CAD build for the part. Positions are in the model's coordinates, mm. Face numbers are marked on the shaded views. A direction names the side the tool comes from. Round coordinates to 2 decimals unless told otherwise and drop trailing zeros. Loops run counter-clockwise (first coordinate to the right, second up) from the corner with the lowest first, then second, coordinate; pieces in that order, holes last. Notation, with made-up numbers: (58.25, -6) - (103.25, -6) arc R10 cw to (103.25, 1) - close; hole circle Ø9 at (69.5, 11.5). An arc over 180 degrees is marked (long way). One line per question, with ' | ' between items.
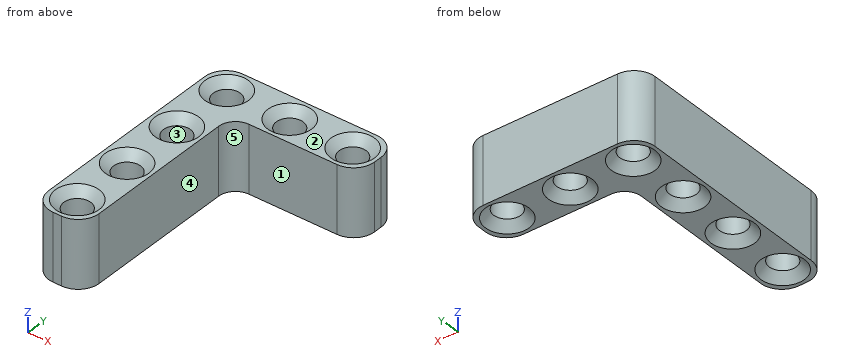
```python
from build123d import *

# Parameters (mm, degrees)
SKETCH1_R           = 1.6
BOSS_EXTRUDE1_DEPTH = 8
CHAMFER1_SIZE       = 1
SKETCH2_R           = 1.6
BOSS_EXTRUDE3_DEPTH = 8
FILLET1_R           = 2
CHAMFER5_SIZE       = 1


with BuildPart() as part:
    # Sketch1 → Boss-Extrude1 (new body)
    with BuildSketch(Plane.XY):
        with BuildLine():
            Line((-0.5, 3), (15.5, 3))
            ThreePointArc((15.5, 3), (17.267766953, 2.267766953), (18, 0.5))
            Line((18, 0.5), (18, -0.5))
            ThreePointArc((18, -0.5), (17.267766953, -2.267766953), (15.5, -3))
            Line((15.5, -3), (-0.5, -3))
            ThreePointArc((-0.5, -3), (-2.267766953, -2.267766953), (-3, -0.5))
            Line((-3, -0.5), (-3, 0.5))
            ThreePointArc((-3, 0.5), (-2.267766953, 2.267766953), (-0.5, 3))
        make_face()
        Circle(SKETCH1_R, mode=Mode.SUBTRACT)
        with Locations((7.5, 0)):
            Circle(SKETCH1_R, mode=Mode.SUBTRACT)
        with Locations((15, 0)):
            Circle(SKETCH1_R, mode=Mode.SUBTRACT)
    extrude(amount=BOSS_EXTRUDE1_DEPTH)

    # Chamfer1
    chamfer1_edges = [part.edges().sort_by_distance(p)[0] for p in [
        (-1.6, 0, 0),
        (-1.6, 0, 8),
        (5.9, 0, 0),
        (5.9, 0, 8),
        (13.4, 0, 0),
        (13.4, 0, 8),
    ]]
    chamfer(chamfer1_edges, length=CHAMFER1_SIZE)

    # Sketch2 → Boss-Extrude3 (add)
    with BuildSketch(Plane.XY.offset(8)):
        with BuildLine():
            ThreePointArc((-0.5, -3), (-2.267766953, -2.267766953), (-3, -0.5))
            Line((-3, -0.5), (-3, -23))
            ThreePointArc((-3, -23), (-2.267766953, -24.767766953), (-0.5, -25.5))
            Line((-0.5, -25.5), (0.5, -25.5))
            ThreePointArc((0.5, -25.5), (2.267766953, -24.767766953), (3, -23))
            Line((3, -23), (3, -3))
            Line((3, -3), (-0.5, -3))
        make_face()
        with Locations((0, -22.5)):
            Circle(SKETCH2_R, mode=Mode.SUBTRACT)
        with Locations((0, -15)):
            Circle(SKETCH2_R, mode=Mode.SUBTRACT)
        with Locations((0, -7.5)):
            Circle(SKETCH2_R, mode=Mode.SUBTRACT)
    extrude(amount=-BOSS_EXTRUDE3_DEPTH)

    # Fillet1
    fillet1_edges = [part.edges().sort_by_distance(p)[0] for p in [
        (3, -3, 4),
    ]]
    fillet(fillet1_edges, radius=FILLET1_R)

    # Chamfer5
    chamfer5_edges = [part.edges().sort_by_distance(p)[0] for p in [
        (-1.6, -7.5, 8),
        (-1.6, -15, 8),
        (-1.6, -22.5, 8),
        (-1.6, -22.5, 0),
        (-1.6, -15, 0),
        (-1.6, -7.5, 0),
    ]]
    chamfer(chamfer5_edges, length=CHAMFER5_SIZE)


solid = part.part
```
(1) Cut at B-B, the plane z = 1.5. Write the cut outline in (x, y).
Results found:
outline: (-3, -23) arc R2.5 ccw to (-0.5, -25.5) - (0.5, -25.5) arc R2.5 ccw to (3, -23) - (3, -5) arc R2 cw to (5, -3) - (15.5, -3) arc R2.5 ccw to (18, -0.5) - (18, 0.5) arc R2.5 ccw to (15.5, 3) - (-0.5, 3) arc R2.5 ccw to (-3, 0.5) - close; hole circle Ø3.2 at (0, -22.5); hole circle Ø3.2 at (0, -15); hole circle Ø3.2 at (0, -7.5); hole circle Ø3.2 at (0, 0); hole circle Ø3.2 at (7.5, 0); hole circle Ø3.2 at (15, 0)
(2) Two-plate mould, pull along Y, no slides. Class the marked faces 3, 4 and 5: released by +Y, released by -Y, zero draft, split by the parting line, or undercut.
Results found:
face 3: undercut | face 4: zero draft | face 5: released by -Y
(3) Tool access for the marked faces 1 and 2: list every direction of +Z, -Z, +X, -X, +Y, -Y with a clear straight run to the whole face (end or side of a thin tool).
Results found:
face 1: +Z, -Z, +X, -Y | face 2: +Z, +X, -X, +Y, -Y
(4) Probe L1, parallel to Y at x = 0, z = 3; L2, parallel to Y at x = 7.5, z = 4.75; L3, parallel to Y at x = 12.5, z = 2.25. List the from-to ranges inside material, lowest first.
Results found:
L1: y = -25.5 to -24.1, -20.9 to -16.6, -13.4 to -9.1, -5.9 to -1.6, 1.6 to 3 | L2: y = -3 to -1.6, 1.6 to 3 | L3: y = -3 to 3
(5) Cut at A-A, the plane y = -22.5. Write the cut outline in (x, z).
Results found:
outline: (-3, 0) - (-2.6, 0) - (-1.6, 1) - (-1.6, 7) - (-2.6, 8) - (-3, 8) - close; (1.6, 1) - (2.6, 0) - (3, 0) - (3, 8) - (2.6, 8) - (1.6, 7) - close
(6) Drop flat-ended pins along their axis: P1, Ø4, axis at x = 0, y = -22.5, coming from the +Z side; P2, Ø3.5, axis at x = 0, y = -7.5, coming from the +Z side; P3, Ø5, axis at x = 0, y = 0, coming from the -Z side; P4, Ø2.5, axis at x = 15, y = 0, coming from the +Z side. Give the stop position or say it passes through.
Results found:
P1: stops at z = 7.4 | P2: stops at z = 7.15 | P3: stops at z = 0.1 | P4: passes through
(7) Cut at C-C, the plane y = 0. Write the cut outline in (x, z), then the cut area to 3 significant figures.
Results found:
outline: (-3, 0) - (-2.6, 0) - (-1.6, 1) - (-1.6, 7) - (-2.6, 8) - (-3, 8) - close; (1.6, 1) - (2.6, 0) - (4.9, 0) - (5.9, 1) - (5.9, 7) - (4.9, 8) - (2.6, 8) - (1.6, 7) - close; (9.1, 1) - (10.1, 0) - (12.4, 0) - (13.4, 1) - (13.4, 7) - (12.4, 8) - (10.1, 8) - (9.1, 7) - close; (16.6, 1) - (17.6, 0) - (18, 0) - (18, 8) - (17.6, 8) - (16.6, 7) - close | area: 85.2 mm²
